Autodesk Fusion 360 part; units mm, degrees
sketch "Sketch1" plane through (0, 0, 0) normal (0, 0, 1) x (1, 0, 0)
  line L0 (0, 0) -> (78, 0)
  line L1 (78, 0) -> (78, 24)
  line L2 (0, 24) -> (0, 0)
  line L3 (12, 12) -> (12, 24) construction
  line L4 (8.5, 15.5707) -> (15.5, 15.5707) construction
  line L5 (8.5, 15.5707) -> (8.5, 24)
  line L6 (15.5, 15.5707) -> (15.5, 24)
  arc A0 (8.5, 15.5707) -> (15.5, 15.5707) centre (12, 12) ccw
  line L7 (8.5, 24) -> (0, 24)
  line L8 (33.5, 15.5707) -> (33.5, 24)
  line L9 (26.5, 15.5707) -> (26.5, 24)
  arc A1 (26.5, 15.5707) -> (33.5, 15.5707) centre (30, 12) ccw
  line L10 (51.5, 15.5707) -> (51.5, 24)
  line L11 (44.5, 15.5707) -> (44.5, 24)
  arc A2 (44.5, 15.5707) -> (51.5, 15.5707) centre (48, 12) ccw
  line L12 (69.5, 15.5707) -> (69.5, 24)
  line L13 (62.5, 15.5707) -> (62.5, 24)
  arc A3 (62.5, 15.5707) -> (69.5, 15.5707) centre (66, 12) ccw
  line L14 (26.5, 24) -> (15.5, 24)
  line L15 (44.5, 24) -> (33.5, 24)
  line L16 (78, 24) -> (69.5, 24)
  line L17 (62.5, 24) -> (51.5, 24)
  dimension "d1" = 10
  dimension "d3" = 12
  dimension "d4" = 12
  dimension "d5" = 3.5
  dimension "d6" = 3.5
  dimension "d7" = 12
  dimension "d10" = 18
  dimension "d11" = 0
  dimension "d12" = 12
extrude "Extrude1" add sketch "Sketch1" along normal blind 9
sketch "Sketch2" plane through (0, 0, 0) normal (-1, 0, 0) x (0, -1, 0)
  line L0 (-24, 0) -> (0, 0)
  line L1 (0, 0) -> (0, 9)
  line L2 (0, 9) -> (-24, 9)
  line L3 (-24, 9) -> (-24, 0)
  line L4 (-24, 9) -> (-16.9844, 9) construction
  line L5 (-18.6, 6) -> (0, 6)
  line L6 (-24, 9) -> (0, 9)
  line L7 (0, 6) -> (0, 9)
  line L8 (-24, 9) -> (-21.6, 9)
  line L9 (-18.6, 6) -> (-21.6, 9)
  dimension "d17" = 3
  dimension "d34" = 45
  dimension "d35" = 2.4
extrude "Extrude2" cut sketch "Sketch2" against normal through all contours L1 L2 L5 L6 L7 L9
sketch "Sketch3" plane through (0, 0, 6) normal (0, 0, 1) x (-1, 0, 0)
  line L0 (-15.5, -18.6) -> (-15.5, -15.5707)
  arc A0 (-8.5, -15.5707) -> (-15.5, -15.5707) centre (-12, -12) ccw
  line L1 (-8.5, -15.5707) -> (-8.5, -18.6)
  line L2 (0, -18.6) -> (0, 0)
  line L3 (0, 0) -> (-78, 0)
  line L4 (-78, 0) -> (-78, -18.6)
  line L5 (-69.5, -18.6) -> (-69.5, -15.5707)
  arc A1 (-62.5, -15.5707) -> (-69.5, -15.5707) centre (-66, -12) ccw
  line L6 (-62.5, -15.5707) -> (-62.5, -18.6)
  line L7 (-51.5, -18.6) -> (-51.5, -15.5707)
  arc A2 (-44.5, -15.5707) -> (-51.5, -15.5707) centre (-48, -12) ccw
  line L8 (-44.5, -15.5707) -> (-44.5, -18.6)
  line L9 (-33.5, -18.6) -> (-33.5, -15.5707)
  arc A3 (-26.5, -15.5707) -> (-33.5, -15.5707) centre (-30, -12) ccw
  line L10 (-26.5, -15.5707) -> (-26.5, -18.6)
  line L11 (0, 0) -> (0, 20)
  line L12 (0, 20) -> (-10, 20)
  line L13 (-10, 20) -> (-21.547, 0)
  line L14 (-78, 0) -> (-78, 20)
  line L15 (-78, 20) -> (-68, 20)
  line L16 (-68, 20) -> (-56.453, 0)
  line L17 (0, 0) -> (-21.547, 0)
  line L18 (-56.453, 0) -> (-78, 0)
  line L19 (-8.5, -18.6) -> (0, -18.6)
  line L20 (-78, -18.6) -> (-69.5, -18.6)
  line L21 (-62.5, -18.6) -> (-51.5, -18.6)
  line L22 (-44.5, -18.6) -> (-33.5, -18.6)
  line L23 (-26.5, -18.6) -> (-15.5, -18.6)
  dimension "d25" = 20
  dimension "d26" = 10
  dimension "d27" = 10
  dimension "d28" = 60
  dimension "d29" = 60
extrude "Extrude3" add sketch "Sketch3" against normal up to surface (6 mm away) contours L3 L11 L12 L13 L17 | L3 L14 L15 L16 L18
sketch "Sketch4" plane through (0, 0, 6) normal (0, 0, 1) x (-1, 0, 0)
  line L0 (-15.5, -18.6) -> (-15.5, -15.5707)
  arc A0 (-8.5, -15.5707) -> (-15.5, -15.5707) centre (-12, -12) ccw
  line L1 (-8.5, -15.5707) -> (-8.5, -18.6)
  line L2 (-8.5, -18.6) -> (0, -18.6)
  line L3 (0, -18.6) -> (0, 20)
  line L4 (0, 20) -> (-10, 20)
  line L5 (-10, 20) -> (-21.547, 0)
  line L6 (-21.547, 0) -> (-56.453, 0)
  line L7 (-56.453, 0) -> (-68, 20)
  line L8 (-68, 20) -> (-78, 20)
  line L9 (-78, 20) -> (-78, -18.6)
  line L10 (-78, -18.6) -> (-69.5, -18.6)
  line L11 (-69.5, -18.6) -> (-69.5, -15.5707)
  arc A1 (-62.5, -15.5707) -> (-69.5, -15.5707) centre (-66, -12) ccw
  line L12 (-62.5, -15.5707) -> (-62.5, -18.6)
  line L13 (-62.5, -18.6) -> (-51.5, -18.6)
  line L14 (-51.5, -18.6) -> (-51.5, -15.5707)
  arc A2 (-44.5, -15.5707) -> (-51.5, -15.5707) centre (-48, -12) ccw
  line L15 (-44.5, -15.5707) -> (-44.5, -18.6)
  line L16 (-44.5, -18.6) -> (-33.5, -18.6)
  line L17 (-33.5, -18.6) -> (-33.5, -15.5707)
  arc A3 (-26.5, -15.5707) -> (-33.5, -15.5707) centre (-30, -12) ccw
  line L18 (-26.5, -15.5707) -> (-26.5, -18.6)
  line L19 (-26.5, -18.6) -> (-15.5, -18.6)
  circle A4 centre (-6.7321, 14) radius 2.25
  line L20 (0, 14) -> (-13.4641, 14) construction
  line L21 (-64.5359, 14) -> (-78, 14) construction
  circle A5 centre (-71.2679, 14) radius 2.25
  dimension "d36" = 4.5
  dimension "d37" = 6
  dimension "d38" = 4.5
extrude "Extrude5" cut sketch "Sketch4" against normal through all contours A4 | A5
fillet "Fillet1" radius 5.5 8 edges at (8.5, 15.5707, 3) (15.5, 15.5707, 3) (26.5, 15.5707, 3) (33.5, 15.5707, 3) (44.5, 15.5707, 3) (51.5, 15.5707, 3) (69.5, 15.5707, 3) (62.5, 15.5707, 3)
fillet "Fillet2" radius 3 10 edges at (69.5, 24, 4.5) (78, 24, 4.5) (62.5, 24, 4.5) (51.5, 24, 4.5) (44.5, 24, 4.5) (33.5, 24, 4.5) (26.5, 24, 4.5) (15.5, 24, 4.5) (8.5, 24, 4.5) (0, 24, 4.5)
fillet "Fillet3" radius 6 6 edges at (0, -20, 3) (10, -20, 3) (21.547, 0, 3) (56.453, 0, 3) (68, -20, 3) (78, -20, 3)
sketch "Sketch5" plane through (0, 0, 6) normal (0, 0, 1) x (-1, 0, 0)
  circle A0 centre (-6.7321, 14) radius 2.25
  circle A1 centre (-71.2679, 14) radius 2.25
  arc A2 (-72, 20) -> (-78, 14) centre (-72, 14) ccw
  line L0 (-78, 14) -> (-78, -18.6)
  line L1 (-78, -18.6) -> (-69.5, -18.6)
  line L2 (-69.5, -18.6) -> (-69.5, -17.4083)
  arc A3 (-69.5, -17.4083) -> (-70.2857, -14.5754) centre (-75, -17.4083) ccw
  arc A4 (-61.7143, -14.5754) -> (-70.2857, -14.5754) centre (-66, -12) ccw
  arc A5 (-61.7143, -14.5754) -> (-62.5, -17.4083) centre (-57, -17.4083) ccw
  line L3 (-62.5, -17.4083) -> (-62.5, -18.6)
  line L4 (-62.5, -18.6) -> (-51.5, -18.6)
  line L5 (-51.5, -18.6) -> (-51.5, -17.4083)
  arc A6 (-51.5, -17.4083) -> (-52.2857, -14.5754) centre (-57, -17.4083) ccw
  arc A7 (-43.7143, -14.5754) -> (-52.2857, -14.5754) centre (-48, -12) ccw
  arc A8 (-43.7143, -14.5754) -> (-44.5, -17.4083) centre (-39, -17.4083) ccw
  line L6 (-44.5, -17.4083) -> (-44.5, -18.6)
  line L7 (-44.5, -18.6) -> (-33.5, -18.6)
  line L8 (-33.5, -18.6) -> (-33.5, -17.4083)
  arc A9 (-33.5, -17.4083) -> (-34.2857, -14.5754) centre (-39, -17.4083) ccw
  arc A10 (-25.7143, -14.5754) -> (-34.2857, -14.5754) centre (-30, -12) ccw
  arc A11 (-25.7143, -14.5754) -> (-26.5, -17.4083) centre (-21, -17.4083) ccw
  line L9 (-26.5, -17.4083) -> (-26.5, -18.6)
  line L10 (-26.5, -18.6) -> (-15.5, -18.6)
  line L11 (-15.5, -18.6) -> (-15.5, -17.4083)
  arc A12 (-15.5, -17.4083) -> (-16.2857, -14.5754) centre (-21, -17.4083) ccw
  arc A13 (-7.7143, -14.5754) -> (-16.2857, -14.5754) centre (-12, -12) ccw
  arc A14 (-7.7143, -14.5754) -> (-8.5, -17.4083) centre (-3, -17.4083) ccw
  line L12 (-8.5, -17.4083) -> (-8.5, -18.6)
  line L13 (-8.5, -18.6) -> (0, -18.6)
  line L14 (0, -18.6) -> (0, 14)
  arc A15 (0, 14) -> (-6, 20) centre (-6, 14) ccw
  line L15 (-6, 20) -> (-6.5359, 20)
  arc A16 (-6.5359, 20) -> (-11.7321, 17) centre (-6.5359, 14) ccw
  line L16 (-11.7321, 17) -> (-19.815, 3)
  arc A17 (-25.0111, 0) -> (-19.815, 3) centre (-25.0111, 6) ccw
  line L17 (-25.0111, 0) -> (-52.9889, 0)
  arc A18 (-58.185, 3) -> (-52.9889, 0) centre (-52.9889, 6) ccw
  line L18 (-58.185, 3) -> (-66.2679, 17)
  arc A19 (-66.2679, 17) -> (-71.4641, 20) centre (-71.4641, 14) ccw
  line L19 (-71.4641, 20) -> (-72, 20)
  line L20 (109.7465, 0) -> (-156.5967, 0)
  line L21 (-156.5967, 0) -> (-156.5967, 57.2242)
  line L22 (-156.5967, 57.2242) -> (109.7465, 57.2242)
  line L23 (109.7465, 57.2242) -> (109.7465, 0)
equation "d6 = d5"
equation "d27 = d26"
equation "d28 = Angular Dimension-2"
equation "d29 = d28"
equation "d34 = Angular Dimension-2"
Source: CAD feature listing. Evaluate the final solid. Frame: model axes, mm. A direction names the side the tool comes from. Coordinates: 2 decimals unless noted, no trailing zeros. Write each loop counter-clockwise with the first axis right and the second up, starting at its lowest first coordinate (ties: lowest second). Pieces come first, ordered by that corner, then holes. Notation, with made-up numbers: M -20,-23.75 L 1,-23.75 A18 cw 1,3.25 Z; hole C -26,49 d2. An arc over 180 degrees is marked long. Use a Markdown table: item, result.
1) First-contact query: pin 1 Ø6 at (x, y) = (12, 12) entering from +Z; pin 2 Ø2 at (x, z) = (17, 5.5) entering from -Y; pin 3 Ø8 at (x, y) = (37.5, 13.5) entering from +Z. Flat tips, straight axial feed; report the tip coordinate or a pass-through.
Conclusion:
| item | result |
|---|---|
| pin 1 | passes through |
| pin 2 | stops at y = -9.61 |
| pin 3 | stops at z = 6 |
2) Section A-A, the plane y = 12. Output: boundary loops of the cut face in (x, z), then the cut area to 3 significant figures.
Conclusion:
| item | result |
|---|---|
| outline | M 0,0 L 7,0 L 7,6 L 0,6 Z; M 17,0 L 25,0 L 25,6 L 17,6 Z; M 35,0 L 43,0 L 43,6 L 35,6 Z; M 53,0 L 61,0 L 61,6 L 53,6 Z; M 71,0 L 78,0 L 78,6 L 71,6 Z |
| area | 228 mm^2 |
3) Section C-C, the plane x = 48. Output: boundary loops of the cut face in (y, z).
Conclusion:
| item | result |
|---|---|
| outline | M 0,0 L 7,0 L 7,6 L 0,6 Z |
4) Mould query, pull axis X, two halves, no side actions, for faces 1 (the flat face through (38, 2, 0)), 2 (the cylindrical face through (51.695, 15.958, 3.042)), 3 (the flat face through (0, 4, 3)). Classes: pulls with the +X half, pulls with the -X half, needs draft (parallel to the pull), parting line crosses it, or undercut.
Conclusion:
| item | result |
|---|---|
| face 1 | needs draft |
| face 2 | undercut |
| face 3 | pulls with the -X half |
5) Section B-B, the plane y = -9. Output: boundary loops of the cut face in (x, z).
Conclusion:
| item | result |
|---|---|
| outline | M 0,0 L 16.35,0 L 16.35,6 L 0,6 Z; M 61.65,0 L 78,0 L 78,6 L 61.65,6 Z |
6) Section D-D, the plane z = 4. Give the number of separate pieces and of enclosed holes in the cut face, then the cut area to 3 significant figures.
Conclusion:
| item | result |
|---|---|
| separate pieces | 1 |
| enclosed holes | 2 |
| area | 1,910 mm^2 |
7) Reachability of faces 4 (the flat face through (57, 23, 9)), 5 (the cylindrical face through (33.695, 15.958, 3.042)), 6 (the flat face through (33.5, 19, 3)) from +Z, -Z, +X, -X, +Y, -Y: full face, straight path, thin tool, end or side. Return the list, or none.
Conclusion:
| item | result |
|---|---|
| face 4 | +Z, +X, -X, +Y, -Y |
| face 5 | +Z, -Z |
| face 6 | +Z, -Z, +Y |
8) Ray query, L1, parallel to X at y = 20, z = 3.5; L2, parallel to X at y = 12, z = 4.55; L3, parallel to X at y = -10.5, z = 4.75. Return the intervals inside material, ascending.
Conclusion:
| item | result |
|---|---|
| L1 | x = 0 to 8.5, 15.5 to 26.5, 33.5 to 44.5, 51.5 to 62.5, 69.5 to 78 |
| L2 | x = 0 to 7, 17 to 25, 35 to 43, 53 to 61, 71 to 78 |
| L3 | x = 0 to 15.48, 62.52 to 78 |
